from build123d import *

# Parameters (mm, degrees)
F0_R     = 8.75
F1_DEPTH = 4
F2_R     = 3.6616494724
F3_DEPTH = 8.5
F5_D     = 3.7973
F5_DEPTH = 8.5
F5_TIP   = 1.1408240143
F6_R     = 2


with BuildPart() as f1:
    # F0 (on Top) → F1 (new body)
    with BuildSketch(Plane.XY):
        Circle(F0_R)
    extrude(amount=F1_DEPTH)

    # F2 (on face) → F3 (join)
    with BuildSketch(Plane.XY.offset(4)):
        Circle(F2_R)
    extrude(amount=F3_DEPTH)

    # F5
    with Locations(Plane.XY.offset(12.5)):
        with Locations((0, 0)):
            Hole(F5_D / 2, depth=F5_DEPTH)
            with Locations((0, 0, -(F5_DEPTH + F5_TIP / 2))):  # 118° drill point
                Cone(0, F5_D / 2, F5_TIP, mode=Mode.SUBTRACT)

    # F6
    f6_edges = [f1.edges().sort_by_distance(p)[0] for p in [
        (-8.75, 0, 0),
    ]]
    fillet(f6_edges, radius=F6_R)


solid = f1.part
The listing builds one solid part. Answer for the finished solid, in the listing's coordinates (mm). A direction names the side the tool comes from. Coordinates: 2 decimals unless noted, no trailing zeros. Loops run counter-clockwise (first coordinate to the right, second up) from the corner with the lowest first, then second, coordinate; pieces in that order, holes last. Notation, with made-up numbers: (9.5, 21.25) -> (68.5, 21.25) arc R20 ccw to (68.5, 49.25) -> close; hole circle Ø4 at (38, -26.5). An arc over 180 degrees is marked (long way). Write item = value, one per line. Start each with the question number.
1) A tool of negligible diameter and unlimited length cuts with its end or side. For faces 1 (the face through (2, -2, 12.5)), 2 (the face through (-2.699, 2.475, 8.19)), from which of +Z, -Z, +X, -X, +Y, -Y can it reach the whole face along a straight path? Write none if from no direction.
2) Straight lines are drawn through the part: line 1 (Y direction, x = 0, z = 7.5); line 2 (Z direction, x = -3.5, y = -4.75); line 3 (Y direction, x = 1.5, z = 8.25). For each, find the intervals that lie inside material, in ascending order. Write a range as from..to.
3) Given pin 1 Ø1.5 at (x, z) = (2.5, 5) entering from +Y; pin 2 Ø2 at (x, z) = (-3.5, 5.5) entering from +Y; pin 3 Ø4.5 at (x, y) = (0, 0) entering from -Z; pin 4 Ø6 at (x, z) = (6, 4) entering from +Y, each flat-ended and moving along its own axis, determine where each tip first touches the part or whether it passes through.
4) A cutting plane is placed at A-A (z = 9.5). Give the vertices of the cut face in (x, y).
5) The mould has two halves that part along Y. Classify faces 3 (the face through (-1.8, 0.6, 8.2)), 4 (the face through (-6.944, -5.324, 2.986)), 5 (the face through (0, 0, 0)): released by +Y, released by -Y, zero draft, split by the parting line, or undercut.
Responses:
q1.face_1 = +Z, +X, -X, +Y, -Y
q1.face_2 = +Z
q2.line_1 = -3.66..-1.9, 1.9..3.66
q2.line_2 = 0..4
q2.line_3 = -3.34..-1.16, 1.16..3.34
q3.pin_1 = 3.22
q3.pin_2 = 2.68
q3.pin_3 = 0
q3.pin_4 = 8.22
q4.outline = circle Ø7.32 at (0, 0); hole circle Ø3.8 at (0, 0)
q5.face_3 = undercut
q5.face_4 = split by the parting line
q5.face_5 = zero draft
